The listing builds one solid part. Answer for the finished solid, in the listing's coordinates (mm). A direction names the side the tool comes from. Give positions to 0.01 mm unless a question says otherwise; leave off trailing zeros. Order: outer loops, then holes, each group sorted by start corner. A loop starts at its lowest first (then second) coordinate and runs counter-clockwise, first axis right, second up. Notation, with made-up numbers: (50.5, 81) - (90.5, 81) arc R24 ccw to (90.5, 97) - close; hole circle Ø11 at (31, 1.5). An arc over 180 degrees is marked (long way). Use a Markdown table: item, result. Add a question column.
1) For faces 1 (the face through (116, -12, -1.6)), 2 (the face through (48, -12, 0)), 3 (the face through (39.777, 10.236, 1.676)), determine the directions among +Z, -Z, +X, -X, +Y, -Y from which every point of the face is accessible in a straight line to the end or side of a thin tool.
2) The mould has two halves that part along X. Classify faces 4 (the face through (79.72, -12.26, -4.65)), 5 (the face through (99, 5, -2)), 6 (the face through (56.313, -3.266, 1.676)): released by +X, released by -X, zero draft, split by the parting line, or undercut.
3) Find section D-D, the plane y = 9.5. Determine the outline of the cut face in (x, z).
4) Straight lines are drawn through the part: line 1 (Z direction, x = 92, y = -16.5); line 2 (Z direction, x = 69, y = -21.5); line 3 (Y direction, x = 99, z = -2.25). For each, find the intervals that lie inside material, in ascending order.
5) Find section A-A, the plane y = -2.5. Determine the outline of the cut face in (x, z), plus the area to 3 significant figures.
6) Flat-ended cylindrical pins translate along their axes: pin 1 (0.5 mm diameter, centred on y = -15.5, z = 2.5, fed in from -X); pin 2 (5 mm diameter, centred on x = 95.5, y = -22.5, fed in from -Z); pin 3 (6.5 mm diameter, centred on x = 43.16, y = -2.5, fed in from -Z); pin 4 (13 mm diameter, centred on x = 96.34, y = -22.5, fed in from -Z). Find the tip coordinate at first contact, or state that the pin passes through.
7) Find section B-B, the plane x = 84.5. Determine the outline of the cut face in (y, z), plus the area to 3 significant figures.
8) Find section C-C, the plane y = -22.5. Determine the outline of the cut face in (x, z).
from build123d import *

# Parameters (mm, degrees)
BOSS_EXTRUDE1_DEPTH = 3.4
SKETCH3_R           = 5
CUT_EXTRUDE1_DEPTH  = 6
CUT_EXTRUDE2_DEPTH  = 10
SKETCH6_R           = 35
CUT_EXTRUDE3_DEPTH  = 10
CUT_EXTRUDE4_DEPTH  = 1
CUT_EXTRUDE5_REACH  = 87.508
SKETCH8_W           = 12
SKETCH8_H           = 35
BOSS_EXTRUDE2_DEPTH = 35
SKETCH10_R          = 4
CUT_EXTRUDE6_DEPTH  = 10
CUT_EXTRUDE7_REACH  = 153.093
SKETCH11_R          = 2
CUT_EXTRUDE8_REACH  = 153.243
SKETCH12_R          = 2


with BuildPart() as part:
    # Sketch1 → Boss-Extrude1 (new body)
    with BuildSketch(Plane.XY):
        with BuildLine():
            Line((0, -30), (80, -30))
            Line((80, -30), (80, 5))
            Line((80, 5), (48, 5))
            Line((48, 5), (16.114075804, 25.304872277))
            ThreePointArc((16.114075804, 25.304872277), (-28.802310396, 8.392074585), (0, -30))
        make_face()
    extrude(amount=BOSS_EXTRUDE1_DEPTH)

    # Sketch3 → Cut-Extrude1 (cut)
    with BuildSketch(Plane.XY.offset(3.4)):
        Circle(SKETCH3_R)
    extrude(amount=-CUT_EXTRUDE1_DEPTH, mode=Mode.SUBTRACT)

    # Sketch5 → Cut-Extrude2 (cut)
    with BuildSketch(Plane.XY.offset(3.4)):
        with BuildLine():
            ThreePointArc((0, 10), (-8.660254038, 5), (-8.660254038, -5))
            ThreePointArc((-8.660254038, -5), (-10.124355653, -10.464101615), (-15.588457268, -9))
            ThreePointArc((-15.588457268, -9), (-15.588457268, 9), (0, 18))
            ThreePointArc((0, 18), (4, 14), (0, 10))
        make_face()
    extrude(amount=-CUT_EXTRUDE2_DEPTH, mode=Mode.SUBTRACT)

    # Sketch6 → Cut-Extrude3 (cut)
    with BuildSketch(Plane(origin=(0, 0, 0), x_dir=(-1, 0, 0), z_dir=(0, 0, -1))):
        Circle(SKETCH6_R)
    extrude(amount=-CUT_EXTRUDE3_DEPTH, mode=Mode.SUBTRACT)

    # Sketch7 → Cut-Extrude4 (cut)
    with BuildSketch(Plane.XY.offset(3.4)):
        Polygon((62.77538264, -13.5), (62.77538264, -20), (64.77538264, -20), (64.77538264, -13.5), (71.27538264, -13.5), (71.27538264, -11.5), (64.77538264, -11.5), (64.77538264, -5), (62.77538264, -5), (62.77538264, -11.5), (56.27538264, -11.5), (56.27538264, -13.5), align=None)
    extrude(amount=-CUT_EXTRUDE4_DEPTH, mode=Mode.SUBTRACT)

    # Sketch8 → Cut-Extrude5 (cut, up to next)
    with BuildSketch(Plane(origin=(0, 0, 0), x_dir=(-1, 0, 0), z_dir=(0, 0, -1)), mode=Mode.PRIVATE) as cut_extrude5_sk1:
        with Locations((-74, -12.5)):
            Rectangle(SKETCH8_W, SKETCH8_H)
    cut_extrude5_tool1 = extrude(cut_extrude5_sk1.sketch, amount=-CUT_EXTRUDE5_REACH, mode=Mode.PRIVATE) & part.part
    add(cut_extrude5_tool1.solids().sort_by_distance((74, -12.5, 0))[0], mode=Mode.SUBTRACT)

    # Sketch9 → Boss-Extrude2 (add)
    with BuildSketch(Plane(origin=(0, 5, 0), x_dir=(1, 0, 0), z_dir=(0, 1, 0))):
        with BuildLine():
            Line((68, 0), (68.320508076, 0))
            ThreePointArc((68.320508076, 0), (70.908698527, 0.340741737), (73.320508076, 1.339745962))
            Line((73.320508076, 1.339745962), (77.339745962, 3.660254038))
            ThreePointArc((77.339745962, 3.660254038), (79.751555511, 4.659258263), (82.339745962, 5))
            Line((82.339745962, 5), (83, 5))
            Line((83, 5), (148, 5))
            Line((148, 5), (148, 1.6))
            Line((148, 1.6), (83, 1.6))
            Line((83, 1.6), (82.339745962, 1.6))
            ThreePointArc((82.339745962, 1.6), (80.631540264, 1.375110454), (79.039745962, 0.715767665))
            Line((79.039745962, 0.715767665), (75.020508076, -1.604740411))
            ThreePointArc((75.020508076, -1.604740411), (71.78868328, -2.943406072), (68.320508076, -3.4))
            Line((68.320508076, -3.4), (68, -3.4))
            Line((68, -3.4), (68, 0))
        make_face()
    extrude(amount=-BOSS_EXTRUDE2_DEPTH)

    # Sketch10 → Cut-Extrude6 (cut)
    with BuildSketch(Plane(origin=(0, 0, -5), x_dir=(-1, 0, 0), z_dir=(0, 0, -1))):
        with Locations((-96.339745962, -2.5)):
            Circle(SKETCH10_R)
        with Locations(Location((-96.339745962, -22.5, 0), (0, 0, 180))):
            Circle(SKETCH10_R)
    extrude(amount=-CUT_EXTRUDE6_DEPTH, mode=Mode.SUBTRACT)

    # Sketch11 → Cut-Extrude7 (cut, up to next)
    with BuildSketch(Plane(origin=(0, 0, 0), x_dir=(-1, 0, 0), z_dir=(0, 0, -1)), mode=Mode.PRIVATE) as cut_extrude7_sk1:
        with Locations((-58.160254038, -22.5)):
            Circle(SKETCH11_R)
    cut_extrude7_tool1 = extrude(cut_extrude7_sk1.sketch, amount=-CUT_EXTRUDE7_REACH, mode=Mode.PRIVATE) & part.part
    # Sketch11 → Cut-Extrude7 (cut, up to next)
    with BuildSketch(Plane(origin=(0, 0, 0), x_dir=(-1, 0, 0), z_dir=(0, 0, -1)), mode=Mode.PRIVATE) as cut_extrude7_sk2:
        with Locations((-58.160254038, -2.5)):
            Circle(SKETCH11_R)
    cut_extrude7_tool2 = extrude(cut_extrude7_sk2.sketch, amount=-CUT_EXTRUDE7_REACH, mode=Mode.PRIVATE) & part.part
    # Sketch11 → Cut-Extrude7 (cut, up to next)
    with BuildSketch(Plane(origin=(0, 0, 0), x_dir=(-1, 0, 0), z_dir=(0, 0, -1)), mode=Mode.PRIVATE) as cut_extrude7_sk3:
        with Locations((-43.160254038, -22.5)):
            Circle(SKETCH11_R)
    cut_extrude7_tool3 = extrude(cut_extrude7_sk3.sketch, amount=-CUT_EXTRUDE7_REACH, mode=Mode.PRIVATE) & part.part
    # Sketch11 → Cut-Extrude7 (cut, up to next)
    with BuildSketch(Plane(origin=(0, 0, 0), x_dir=(-1, 0, 0), z_dir=(0, 0, -1)), mode=Mode.PRIVATE) as cut_extrude7_sk4:
        with Locations((-43.160254038, -2.5)):
            Circle(SKETCH11_R)
    cut_extrude7_tool4 = extrude(cut_extrude7_sk4.sketch, amount=-CUT_EXTRUDE7_REACH, mode=Mode.PRIVATE) & part.part
    add(cut_extrude7_tool1.solids().sort_by_distance((58.160254, -22.5, 0))[0], mode=Mode.SUBTRACT)
    add(cut_extrude7_tool2.solids().sort_by_distance((58.160254, -2.5, 0))[0], mode=Mode.SUBTRACT)
    add(cut_extrude7_tool3.solids().sort_by_distance((43.160254, -22.5, 0))[0], mode=Mode.SUBTRACT)
    add(cut_extrude7_tool4.solids().sort_by_distance((43.160254, -2.5, 0))[0], mode=Mode.SUBTRACT)

    # Sketch12 → Cut-Extrude8 (cut, up to next)
    with BuildSketch(Plane(origin=(0, 0, -5), x_dir=(-1, 0, 0), z_dir=(0, 0, -1)), mode=Mode.PRIVATE) as cut_extrude8_sk1:
        with Locations((-116.339745962, -22.5)):
            Circle(SKETCH12_R)
    cut_extrude8_tool1 = extrude(cut_extrude8_sk1.sketch, amount=-CUT_EXTRUDE8_REACH, mode=Mode.PRIVATE) & part.part
    # Sketch12 → Cut-Extrude8 (cut, up to next)
    with BuildSketch(Plane(origin=(0, 0, -5), x_dir=(-1, 0, 0), z_dir=(0, 0, -1)), mode=Mode.PRIVATE) as cut_extrude8_sk2:
        with Locations((-116.339745962, -2.5)):
            Circle(SKETCH12_R)
    cut_extrude8_tool2 = extrude(cut_extrude8_sk2.sketch, amount=-CUT_EXTRUDE8_REACH, mode=Mode.PRIVATE) & part.part
    add(cut_extrude8_tool1.solids().sort_by_distance((116.339746, -22.5, -5))[0], mode=Mode.SUBTRACT)
    add(cut_extrude8_tool2.solids().sort_by_distance((116.339746, -2.5, -5))[0], mode=Mode.SUBTRACT)


solid = part.part
The answers:
| question | item | result |
|---|---|---|
| 1 | face 1 | +Z, +X, +Y, -Y |
| 1 | face 2 | -Z, -X, +Y, -Y |
| 1 | face 3 | +Z, -Z, +X, +Y |
| 2 | face 4 | released by -X |
| 2 | face 5 | zero draft |
| 2 | face 6 | undercut |
| 3 | outline | (33.69, 0) - (40.93, 0) - (40.93, 3.4) - (33.69, 3.4) - close |
| 4 | line 1 | -5 to -1.6 |
| 4 | line 2 | -0.02 to 3.38 |
| 4 | line 3 | -30 to -25.49, -19.51 to -5.49, 0.49 to 5 |
| 5 | outline | (34.91, 0) - (41.16, 0) - (41.16, 3.4) - (34.91, 3.4) - close; (45.16, 0) - (56.16, 0) - (56.16, 3.4) - (45.16, 3.4) - close; (60.16, 0) - (68.32, 0) arc R10 cw to (73.32, -1.34) - (77.34, -3.66) arc R10 ccw to (82.34, -5) - (92.34, -5) - (92.34, -1.6) - (82.34, -1.6) arc R6.6 cw to (79.04, -0.72) - (75.02, 1.6) arc R13.4 ccw to (68.32, 3.4) - (60.16, 3.4) - close; (100.34, -5) - (114.34, -5) - (114.34, -1.6) - (100.34, -1.6) - close; (118.34, -5) - (148, -5) - (148, -1.6) - (118.34, -1.6) - close |
| 5 | area | 320 mm2 |
| 6 | pin 1 | x = 31.26 |
| 6 | pin 2 | through |
| 6 | pin 3 | z = 0 |
| 6 | pin 4 | z = -5 |
| 7 | outline | (-30, -5) - (5, -5) - (5, -1.6) - (-30, -1.6) - close |
| 7 | area | 119 mm2 |
| 8 | outline | (26.81, 0) - (41.16, 0) - (41.16, 3.4) - (26.81, 3.4) - close; (45.16, 0) - (56.16, 0) - (56.16, 3.4) - (45.16, 3.4) - close; (60.16, 0) - (68.32, 0) arc R10 cw to (73.32, -1.34) - (77.34, -3.66) arc R10 ccw to (82.34, -5) - (92.34, -5) - (92.34, -1.6) - (82.34, -1.6) arc R6.6 cw to (79.04, -0.72) - (75.02, 1.6) arc R13.4 ccw to (68.32, 3.4) - (60.16, 3.4) - close; (100.34, -5) - (114.34, -5) - (114.34, -1.6) - (100.34, -1.6) - close; (118.34, -5) - (148, -5) - (148, -1.6) - (118.34, -1.6) - close |
